The drawing under review shows one solid part. Ordinate dimensions are in mm from its lowest x, y, z. A direction names the side the tool comes from. Coordinates: 2 decimals unless noted, no trailing zeros. Order: outer loops, then holes, each group sorted by start corner. A loop starts at its lowest first (then second) coordinate and runs counter-clockwise, first axis right, second up.
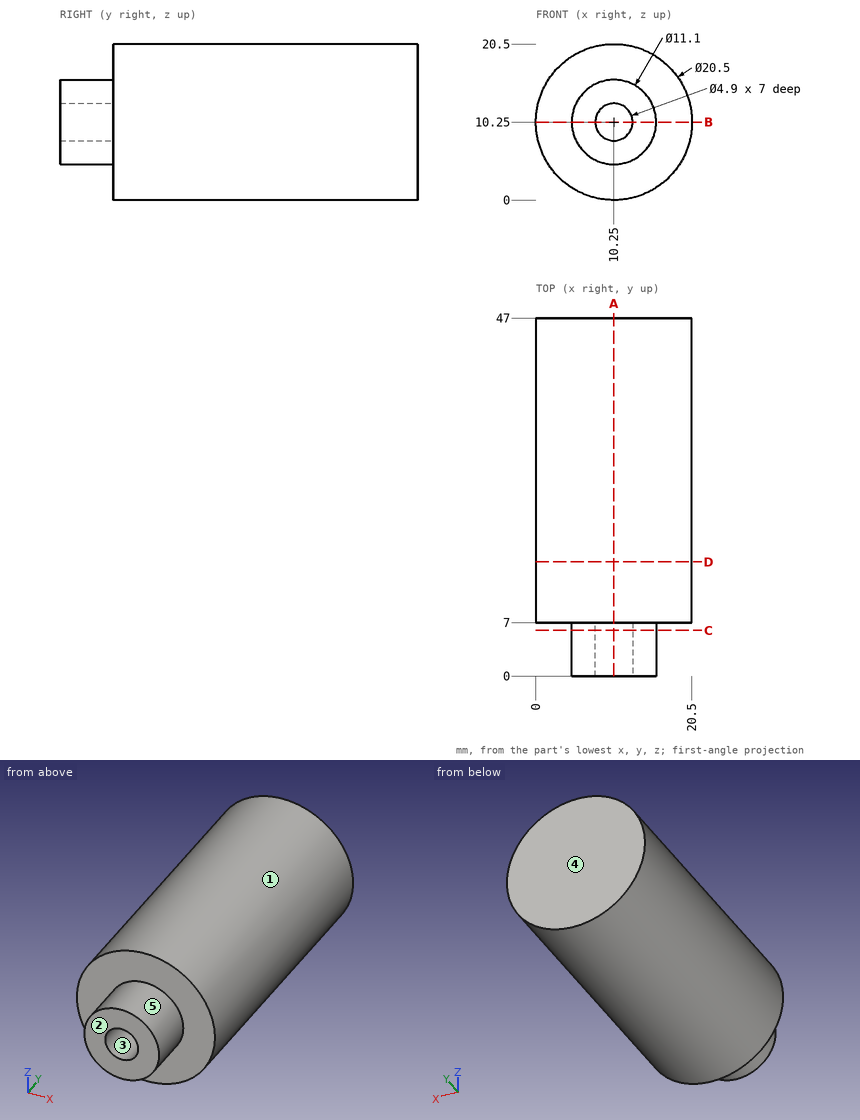
1. Mouldability with a two-part tool opening along Z and no side actions: class the marked faces 1, 2 and 3 as pulls with the +Z half, pulls with the -Z half, needs draft (parallel to the pull), parting line crosses it, or undercut.
2. To check wall thickness, follow line 1 (Z direction, x = 10.25, y = 5.75); line 2 (Y direction, x = 18.25, z = 7.75); line 3 (Z direction, x = 6, y = 33). State the ranges of each line that lie inside material, in increasing order.
3. For the marked faces 4 and 5, list the 3-axis set-ups (+Z, -Z, +X, -X, +Y, -Y) from which the entire face can be reached by the end or side of a thin tool; tool diameter is ignored.
4. Add section C-C (y = 6). Give the boundary of the cut face in (x, z), and give its area (3 significant figures).
5. Add section D-D (y = 15). Give the boundary of the cut face in (x, z), and give its area (3 significant figures).
6. Add section A-A (x = 10.25). Give the boundary of the cut face in (y, z).
7. Insertion check: pin 1 (2 mm diameter, centred on x = 4.5, y = 19.5, fed in from -Z); pin 2 (6 mm diameter, centred on x = 4, y = 27.5, fed in from -Z); pin 3 (3 mm diameter, centred on y = 42, z = 17, fed in from +X). Each pin has a flat end and moves straight along its axis. Give the tip position at first contact, or say it passes through.
8. Add section B-B (z = 10.25). Give the boundary of the cut face in (x, y).
Solution:
1. face 1: parting line crosses it
1. face 2: needs draft
1. face 3: undercut
2. line 1: z = 4.7 to 7.8, 12.7 to 15.8
2. line 2: y = 7 to 47
2. line 3: z = 0.92 to 19.58
3. face 4: +Z, -Z, +X, -X, +Y
3. face 5: -Y
4. outline: circle Ø11.1 at (10.25, 10.25); hole circle Ø4.9 at (10.25, 10.25)
4. area: 77.9 mm2
5. outline: circle Ø20.5 at (10.25, 10.25)
5. area: 330 mm2
6. outline: (0, 4.7) - (7, 4.7) - (7, 0) - (47, 0) - (47, 20.5) - (7, 20.5) - (7, 15.8) - (0, 15.8) - (0, 12.7) - (7, 12.7) - (7, 7.8) - (0, 7.8) - close
7. pin 1: stops at z = 1.17
7. pin 2: stops at z = 0.53
7. pin 3: stops at x = 19.05
8. outline: (0, 7) - (4.7, 7) - (4.7, 0) - (7.8, 0) - (7.8, 7) - (12.7, 7) - (12.7, 0) - (15.8, 0) - (15.8, 7) - (20.5, 7) - (20.5, 47) - (0, 47) - close
